Can you work these out from the model? Positions are in its coordinate system, mm. Face numbers are marked on the shaded views. Round coordinates to 2 decimals unless told otherwise and drop trailing zeros. Loops run counter-clockwise (first coordinate to the right, second up) from the corner with the lowest first, then second, coordinate; pieces in that order, holes last. Notation, with made-up numbers: (-17.75, 37) - (5.25, 37) arc R8 ccw to (5.25, 50) - close; hole circle Ø5 at (-20.75, 15). An arc over 180 degrees is marked (long way). Answer as CSV lines item,"result".
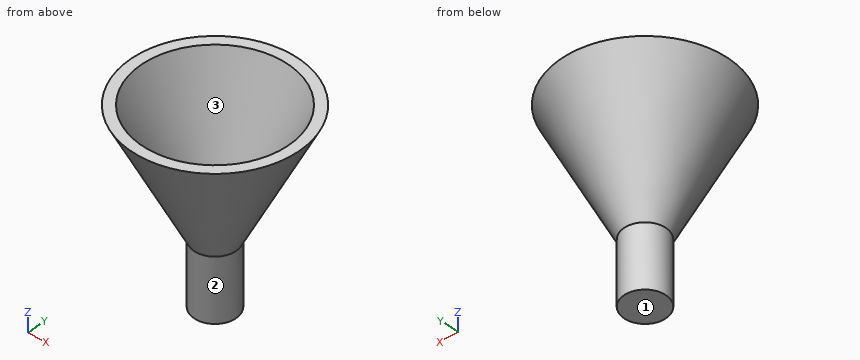
```python
from build123d import *

# Parameters (mm, degrees)
CYLINDER_R        = 1
CYLINDER_DEPTH    = 3
CYLINDER001_R     = 0.5
CYLINDER001_DEPTH = 3


with BuildPart() as cone001:
    # Cone001 → Cone001 (revolve)
    with BuildSketch(Plane(origin=(0, 0, 3), x_dir=(1, 0, 0), z_dir=(0, -1, 0))):
        Polygon((0, 0), (0.5, 0), (3.5, 6), (0, 6), align=None)
    revolve(axis=Axis((0, 0, 3), (0, 0, 1)))


with BuildPart() as cut001:
    # Cone → Cone (revolve)
    with BuildSketch(Plane(origin=(0, 0, 3), x_dir=(1, 0, 0), z_dir=(0, -1, 0))):
        Polygon((0, 0), (1, 0), (4, 6), (0, 6), align=None)
    revolve(axis=Axis((0, 0, 3), (0, 0, 1)))

    # Cut001: cut Cone001
    add(cone001.part, mode=Mode.SUBTRACT)


with BuildPart() as cylinder:
    # Cylinder → Cylinder (new body)
    with BuildSketch(Plane.XY):
        Circle(CYLINDER_R)
    extrude(amount=CYLINDER_DEPTH)


with BuildPart() as cylinder001:
    # Cylinder001 → Cylinder001 (new body)
    with BuildSketch(Plane.XY):
        Circle(CYLINDER001_R)
    extrude(amount=CYLINDER001_DEPTH)


with BuildPart() as fusion:
    # Cut base: copy of Cylinder
    add(cylinder.part)

    # Cut: cut Cylinder001
    add(cylinder001.part, mode=Mode.SUBTRACT)

    # Fusion: union Cut001, Cylinder, Cylinder001
    add(cut001.part)
    add(cylinder.part)
    add(cylinder001.part)


solid = fusion.part
```
Q1. We'd pull the mould along Y, two halves only. Please class the marked faces 1, 2 and 3: pulls with the +Y half, pulls with the -Y half, needs draft (parallel to the pull), parting line crosses it, or undercut.
Checks:
face 1,"needs draft"
face 2,"parting line crosses it"
face 3,"undercut"
Q2. I'm going to push flat-ended pins straight in: pin 1 Ø0.8 at (x, y) = (0, 0) entering from +Z; pin 2 Ø1.5 at (x, y) = (3, -0.5) entering from -Z; pin 3 Ø3 at (x, z) = (1, 3.5) entering from +Y. Where does each tip first touch, or does it pass through?
Checks:
pin 1,"z = 3"
pin 2,"z = 5.58"
pin 3,"y = 1.9"
Q3. Imagine slicing it at C-C (z = 2). Write out the boundary of the cut face in (x, y).
Checks:
outline,"circle Ø2 at (0, 0)"
Q4. If I drill on line 1 along X through (y, z) = (1.75, 6.75); line 2 along X through (y, z) = (0.5, 6.25); line 3 along Y through (x, z) = (2.5, 7.5), over which ranges is the centre line in solid material (lowest first)? Write a range as [from, to].
Checks:
line 1,"[-2.28, -1.61], [1.61, 2.28]"
line 2,"[-2.58, -2.07], [2.07, 2.58]"
line 3,"[-2.08, -1.15], [1.15, 2.08]"
Q5. Imagine slicing it at A-A (x = 0). Write out the boundary of the cut face in (y, z).
Checks:
outline,"(-4, 9) - (-1, 3) - (-1, 0) - (1, 0) - (1, 3) - (4, 9) - (3.5, 9) - (0.5, 3) - (-0.5, 3) - (-3.5, 9) - close"
Q6. Imagine slicing it at D-D (z = 5.25). Write out the boundary of the cut face in (x, y) (3 decimals), then the cut area to 3 significant figures.
Checks:
outline,"circle Ø4.25 at (0, 0); hole circle Ø3.25 at (0, 0)"
area,"5.89 mm²"
